Solid Edge part; units mm, degrees
sketch "Sketch1" plane through (0, 0, 0) normal (0, -1, 0) x (1, 0, 0)
  circle A0 centre (0, 0) radius 6
extrude "Protrusion1" add sketch "Sketch1" along normal blind 3.6
sketch "Sketch2" plane through (0, -3.6, 0) normal (0, -1, 0) x (1, 0, 0)
  circle A0 centre (0, 0) radius 3
extrude "Protrusion2" add sketch "Sketch2" along normal blind 16
cosmetic_thread "Thread1"
sketch "Sketch3" plane through (0, 0, 0) normal (0, 1, 0) x (0, 0, -1)
  line L0 (2.5, -1.4434) -> (2.5, 1.4434)
  line L1 (2.5, 1.4434) -> (0, 2.8868)
  line L2 (0, 2.8868) -> (-2.5, 1.4434)
  line L3 (-2.5, 1.4434) -> (-2.5, -1.4434)
  line L4 (-2.5, -1.4434) -> (0, -2.8868)
  line L5 (0, -2.8868) -> (2.5, -1.4434)
extrude "ExtrudedCutout_4" cut sketch "Sketch3" against normal blind 3
chamfer "Chamfer_1" distance 0.15 angle 45 1 edges at (-6, 0, 0)
properties material "Nylon, general purpose"
Input: part model. Units: mm. Frame: model coordinates. A direction names the side the tool comes from. Give positions to 0.01 mm unless a question says otherwise; leave off trailing zeros. Write each loop counter-clockwise with the first axis right and the second up, starting at its lowest first coordinate (ties: lowest second). Pieces come first, ordered by that corner, then holes.
Q1. Material intervals for probe 1 along Y at (x, z) = (2, -2.5); probe 2 along Y at (x, z) = (-1.5, -1.75); probe 3 along X at (y, z) = (-2, 1), sorted ascending.
Q2. Section B-B, the plane y = -16. Output: boundary loops of the cut face in (x, z).
Q3. Section A-A, the plane x = 0. Output: boundary loops of the cut face in (y, z).
Q4. Pull-direction query (Z, two-part tool) for faces 4 (the face through (-3, -11, 0)), 5 (the face through (0, -3, 0)), 6 (the face through (0, 0, -3)); classes: pulls with the +Z half, pulls with the -Z half, needs draft (parallel to the pull), parting line crosses it, or undercut.
Q5. Set-up query: faces 1 (the face through (2.155, -1.479, 1.267)), 2 (the face through (-6, -2, 0)), 3 (the face through (-1, -3.6, 3)). Return all of +Z, -Z, +X, -X, +Y, -Y with unobstructed straight access to the full face (end or side cutting, diameter ignored); none if empty.
Q6. First-contact query: P1, Ø1, axis at y = -2.5, z = -2.5, coming from the -X side; P2, Ø5, axis at y = -9.5, z = -0.5, coming from the +X side; P3, Ø2.5, axis at x = 1, z = 0.5, coming from the +Y side. Flat tips, straight axial feed; report the tip coordinate or a pass-through.
Filled in:
1. probe 1: y = -3.6 to 0
1. probe 2: y = -19.6 to -3
1. probe 3: x = -5.92 to -2.31, 2.31 to 5.92
2. outline: circle Ø6 at (0, 0)
3. outline: (-19.6, -3) - (-3.6, -3) - (-3.6, -6) - (-0.15, -6) - (0, -5.85) - (0, -2.5) - (-3, -2.5) - (-3, 2.5) - (0, 2.5) - (0, 5.85) - (-0.15, 6) - (-3.6, 6) - (-3.6, 3) - (-19.6, 3) - close
4. face 4: parting line crosses it
4. face 5: undercut
4. face 6: needs draft
5. face 1: +Y
5. face 2: +Y, -Y
5. face 3: -Y
6. P1: stops at x = -5.66
6. P2: stops at x = 3
6. P3: stops at y = -3
